from build123d import *

# Parameters (mm, degrees)
BOSS_EXTRUDE1_DEPTH = 150
SKETCH4_R           = 1.65
CUT_EXTRUDE1_DEPTH  = 7
SKETCH5_W           = 1.5
SKETCH5_H           = 150
CUT_EXTRUDE2_DEPTH  = 1


with BuildPart() as part:
    # Sketch1 → Boss-Extrude1 (new body)
    with BuildSketch(Plane.XY):
        Polygon((-75.5, 3.5), (75.5, 3.5), (75.5, -3.5), (23.2, -3.5), (23.2, -13.5), (17.2, -13.5), (17.2, -3.5), (-17.2, -3.5), (-17.2, -13.5), (-23.2, -13.5), (-23.2, -3.5), (-75.5, -3.5), align=None)
    extrude(amount=BOSS_EXTRUDE1_DEPTH)

    # Sketch4 → Cut-Extrude1 (cut)
    with BuildSketch(Plane.XZ.offset(3.5)):
        with Locations((-10, 6)):
            Circle(SKETCH4_R)
        with Locations((10, 6)):
            Circle(SKETCH4_R)
        with Locations((-10, 144)):
            Circle(SKETCH4_R)
        with Locations((10, 144)):
            Circle(SKETCH4_R)
    extrude(amount=-CUT_EXTRUDE1_DEPTH, mode=Mode.SUBTRACT)

    # Sketch5 → Cut-Extrude2 (cut)
    with BuildSketch(Plane(origin=(0, 3.5, 0), x_dir=(1, 0, 0), z_dir=(0, 1, 0))):
        with Locations((-44.75, -75)):
            Rectangle(SKETCH5_W, SKETCH5_H)
        with Locations((-14.75, -75)):
            Rectangle(SKETCH5_W, SKETCH5_H)
        with Locations((15.25, -75)):
            Rectangle(SKETCH5_W, SKETCH5_H)
        with Locations((45.25, -75)):
            Rectangle(SKETCH5_W, SKETCH5_H)
    extrude(amount=-CUT_EXTRUDE2_DEPTH, mode=Mode.SUBTRACT)


solid = part.part
Read the model definition and answer for the solid it produces. Units are mm, in the model's axes. A direction names the side the tool comes from. Coordinates: 2 decimals unless noted, no trailing zeros. Loops run counter-clockwise (first coordinate to the right, second up) from the corner with the lowest first, then second, coordinate; pieces in that order, holes last.
Q1. The mould has two halves that part along X. Classify faces 4 (the face through (-23.2, -9, 74)), 5 (the face through (50, -3.5, 74)), 6 (the face through (0, -3.5, 74)): +X half, -X half, draft (parallel to the pull), parting line (faces both ways), or undercut.
Q2. This flat-tipped pin is pushed along its axis until it touches: pin 1 Ø10 at (y, z) = (-11, 66) entering from +X. Where does it stop, or does it pass through?
Q3. Consider probe 1 along Z at (x, y) = (10, 0.5); probe 2 along X at (y, z) = (-1.25, 144); probe 3 along X at (y, z) = (-5.5, 62). Determine where each line is inside the solid, lowest interval first.
Q4. The part is cut by section C-C on x = -40. Write down the section's boundary in (y, z), and give its area (3 significant figures).
Q5. Which of the six approach directions +Z, -Z, +X, -X, +Y, -Y give full straight-line access (tool end or side, diameter ignored) to faces 1 (the face through (23.2, -8, 74)), 2 (the face through (30, 3.5, 74)), 3 (the face through (-49, -3.5, 74))?
Q6. The part is cut by section A-A on y = -8.25. Write down the section's boundary in (x, z).
Q7. The part is cut by section B-B on z = 105. Write down the section's boundary in (x, y), and give its area (3 significant figures).
Results below:
1. face 4: -X half
1. face 5: draft
1. face 6: undercut
2. pin 1: stops at x = 23.2
3. probe 1: z = 0 to 4.35, 7.65 to 142.35, 145.65 to 150
3. probe 2: x = -75.5 to -11.65, -8.35 to 8.35, 11.65 to 75.5
3. probe 3: x = -23.2 to -17.2, 17.2 to 23.2
4. outline: (-3.5, 0) - (3.5, 0) - (3.5, 150) - (-3.5, 150) - close
4. area: 1,050 mm2
5. face 1: +Z, -Z, +X, -Y
5. face 2: +Z, -Z, +X, -X, +Y
5. face 3: +Z, -Z, -X, -Y
6. outline: (-23.2, 0) - (-17.2, 0) - (-17.2, 150) - (-23.2, 150) - close; (17.2, 0) - (23.2, 0) - (23.2, 150) - (17.2, 150) - close
7. outline: (-75.5, -3.5) - (-23.2, -3.5) - (-23.2, -13.5) - (-17.2, -13.5) - (-17.2, -3.5) - (17.2, -3.5) - (17.2, -13.5) - (23.2, -13.5) - (23.2, -3.5) - (75.5, -3.5) - (75.5, 3.5) - (46, 3.5) - (46, 2.5) - (44.5, 2.5) - (44.5, 3.5) - (16, 3.5) - (16, 2.5) - (14.5, 2.5) - (14.5, 3.5) - (-14, 3.5) - (-14, 2.5) - (-15.5, 2.5) - (-15.5, 3.5) - (-44, 3.5) - (-44, 2.5) - (-45.5, 2.5) - (-45.5, 3.5) - (-75.5, 3.5) - close
7. area: 1,170 mm2
